Design review of the part built by this model. Coordinates are the model's own, in mm. Coordinates: 2 decimals unless noted, no trailing zeros. Write each loop counter-clockwise with the first axis right and the second up, starting at its lowest first coordinate (ties: lowest second). Pieces come first, ordered by that corner, then holes.
Q1. Take a section at B-B, the plane z = 12. Write out the cut boundary in (x, y), plus the area to 3 significant figures.
Q2. For pin 1 Ø1.5 at (y, z) = (5, 22.5) entering from -X, flat-tipped, find the tip position at first contact; note if it passes through.
Q3. For L1, parallel to Z at x = 18.25, y = 1; L2, parallel to Z at x = 14, y = 5.75; L3, parallel to Y at x = 15.75, z = 21, list the stretches that pass through material, from the lowest coordinate up.
Q4. Take a section at D-D, the plane z = 39.5. Write out the cut boundary in (x, y) (3 decimals), plus the area to 3 significant figures.
Q5. Take a section at C-C, the plane y = 6. State how many separate pieces and enclosed holes the cut face has, plus the area to 3 significant figures.
Q6. Take a section at A-A, the plane y = 2.5. Write out the cut boundary in (x, z), plus the area to 3 significant figures.
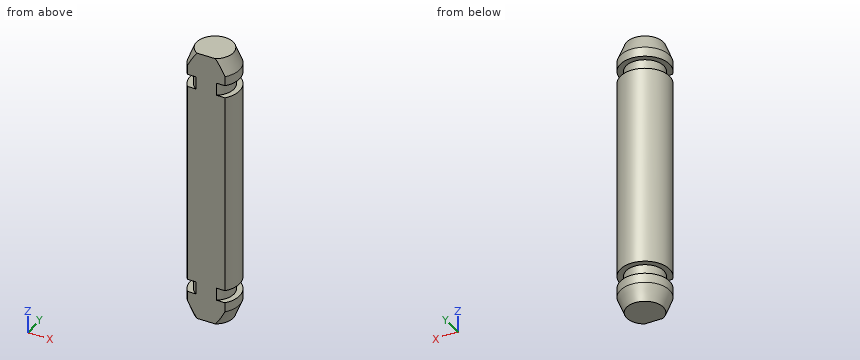
Autodesk Fusion 360 part; units mm, degrees
sketch "Sketch1" plane through (0, 0, 0) normal (0, 0, 1) x (1, 0, 0)
  line L0 (0, 0) -> (5.9867, 0)
  arc A0 (5.9867, 0) -> (0, 0) centre (2.9933, 2.5) ccw
  arc A1 (4.6516, 0) -> (1.335, 0) centre (2.9933, 2.5) ccw
  arc A2 (17.1516, 0) -> (13.835, 0) centre (15.4933, 2.5) ccw
  line L1 (12.5, 0) -> (18.4867, 0)
  arc A3 (18.4867, 0) -> (12.5, 0) centre (15.4933, 2.5) ccw
  arc A4 (29.6516, 0) -> (26.335, 0) centre (27.9933, 2.5) ccw
  line L2 (25, 0) -> (30.9867, 0)
  arc A5 (30.9867, 0) -> (25, 0) centre (27.9933, 2.5) ccw
  point P0 (12.5, 0)
  point P1 (25, 0)
  dimension "d1" = 3.9
  dimension "d2" = 2.5
  dimension "d13" = 6
  dimension "d16" = 25
  dimension "d17" = 0
extrude "Extrude1" add sketch "Sketch1" along normal blind 102 contours L0 A0 A1 | L0 A1 makes body 1
extrude "Extrude2" cut sketch "Sketch1" against normal blind 2 from surface at 6 contours L0 A0 A1 bodies 1
ref_plane "WorkPlane1" through (2.9933, 3.9289, 51) normal (0, 0, 1) x (1, 0, 0)
mirror "Mirror1" about plane through (2.9933, 3.9289, 51) normal (0, 0, 1) of "Extrude2"
extrude "Extrude3" add sketch "Sketch1" along normal blind 44 separate body contours A2 L1 | A2 L1 A3 makes body 2
extrude "Extrude4" cut sketch "Sketch1" against normal blind 2 from surface at 6 contours A2 L1 A3 bodies 2
ref_plane "WorkPlane2" through (15.4933, 3.9289, 22) normal (0, 0, 1) x (1, 0, 0)
mirror "Mirror2" about plane through (15.4933, 3.9289, 22) normal (0, 0, 1) of "Extrude4"
chamfer "Chamfer3" distance 2.5 distance2 1 1 edges at (15.4933, 6.4, 0) measured on face at (12.3817, 0.1488, 2.6667) on bodies 1 2
chamfer "Chamfer3" distance 2.5 distance2 1 1 edges at (2.9933, 6.4, 0) measured on face at (-0.1183, 0.1488, 2.6667) on bodies 1 2
chamfer "Chamfer3" distance 1 distance2 2.5 2 edges at (15.4933, 6.4, 44) (2.9933, 6.4, 102) measured on face at (16.772, 1.0681, 44) measured on face at (3.5688, 2.2017, 102) on bodies 1 2
hidden bodies 1
equation "d7 = Long_Pin + End_Thickness * 2"
equation "C_Clip_Thickness = 2 mm"
equation "End_Thickness = 4 mm + C_Clip_Thickness"
equation "Long_Pin = 90 mm"
equation "Short_Pin = 32 mm"
equation "d18 = End_Thickness"
equation "d25 = Short_Pin + End_Thickness * 2"
equation "d27 = End_Thickness"
Responses:
1. outline: (12.5, 0) - (18.49, 0) arc R3.9 ccw (long way) to start
1. area: 42.0 mm2
2. pin 1: stops at x = 12.01
3. L1: z = 0.6 to 4, 6 to 38, 40 to 43.4
3. L2: z = 1.69 to 4, 6 to 38, 40 to 42.31
3. L3: y = 0 to 6.39
4. outline: (13.835, 0) - (17.152, 0) arc R3 ccw (long way) to start
4. area: 27.1 mm2
5. separate pieces: 3
5. enclosed holes: 0
5. area: 125 mm2
6. outline: (11.59, 2.5) - (12.59, 0) - (18.39, 0) - (19.39, 2.5) - (19.39, 4) - (18.49, 4) - (18.49, 6) - (19.39, 6) - (19.39, 38) - (18.49, 38) - (18.49, 40) - (19.39, 40) - (19.39, 41.5) - (18.39, 44) - (12.59, 44) - (11.59, 41.5) - (11.59, 40) - (12.49, 40) - (12.49, 38) - (11.59, 38) - (11.59, 6) - (12.49, 6) - (12.49, 4) - (11.59, 4) - close
6. area: 331 mm2
